For this review, take the finished solid that the model builds, in its own axes (mm). Face numbers are marked on the shaded views. A direction names the side the tool comes from. Round coordinates to 2 decimals unless told otherwise and drop trailing zeros. Write each loop counter-clockwise with the first axis right and the second up, starting at its lowest first coordinate (ties: lowest second). Pieces come first, ordered by that corner, then holes. Notation, with made-up numbers: (1, 30.5) -> (21, 30.5) arc R12 ccw to (21, 46.5) -> close; hole circle Ø10 at (-3, -32). An arc over 180 degrees is marked (long way). Answer in a Markdown table with one row per item.
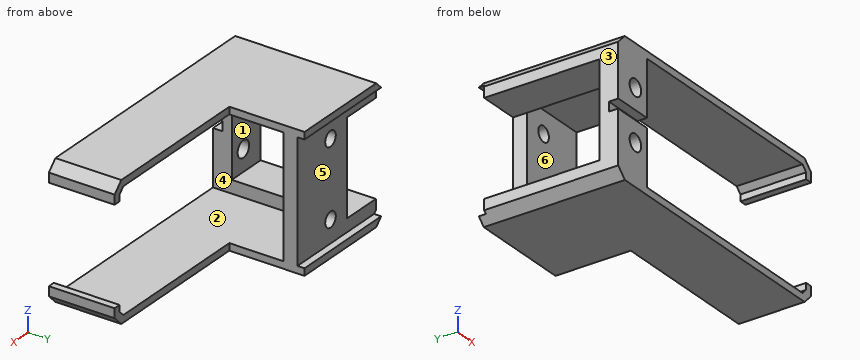
from build123d import *

# Parameters (mm, degrees)
SZKIC1_W                      = 8.7
SZKIC1_H                      = 9
SZKIC1_R                      = 1.75
DODANIE_WYCI_GNI_CIE1_DEPTH   = 2
DODANIE_WYCI_GNI_CIE1_2_DEPTH = 2
SZKIC2_W                      = 8.7
SZKIC2_H                      = 20
SZKIC2_R                      = 1.75
DODANIE_WYCI_GNI_CIE2_DEPTH   = 2
DODANIE_WYCI_GNI_CIE3_DEPTH   = 14
WYTNIJ_WYCI_GNI_CIE1_REACH    = 46.443
DODANIE_WYCI_GNI_CIE7_DEPTH   = 14.5
SZKIC10_W                     = 15
SZKIC10_H                     = 25.5
SZKIC10_R                     = 1.6
DODANIE_WYCI_GNI_CIE9_DEPTH   = 3
DODANIE_WYCI_GNI_CIE10_DEPTH  = 1.5


with BuildPart() as part:
    # Szkic1 → Dodanie-wyci_gni_cie1 (new body)
    with BuildSketch(Plane(origin=(0, 0, 0), x_dir=(1, 0, 0), z_dir=(0, 1, 0))):
        with Locations((-35.35, 5.5)):
            Rectangle(SZKIC1_W, SZKIC1_H)
        with Locations(Location((-34.5, 5.45, 0), (0, 0, 270))):
            Circle(SZKIC1_R, mode=Mode.SUBTRACT)
    extrude(amount=DODANIE_WYCI_GNI_CIE1_DEPTH)



with BuildPart() as body_2:
    # Szkic1 → Dodanie-wyci_gni_cie1 2 (new body)
    with BuildSketch(Plane(origin=(0, 0, 0), x_dir=(1, 0, 0), z_dir=(0, 1, 0))):
        with Locations((-35.35, -5.5)):
            Rectangle(SZKIC1_W, SZKIC1_H)
        with Locations(Location((-34.5, -5.45, 0), (0, 0, 90))):
            Circle(SZKIC1_R, mode=Mode.SUBTRACT)
    extrude(amount=DODANIE_WYCI_GNI_CIE1_2_DEPTH)


with BuildPart() as part_1:
    add(part.part)

    add(body_2.part)  # Dodanie-wyci_gni_cie2 merges body 2
    # Szkic2 → Dodanie-wyci_gni_cie2 (add)
    with BuildSketch(Plane(origin=(0, 2, 0), x_dir=(1, 0, 0), z_dir=(0, 1, 0))):
        with Locations((-35.35, 0)):
            Rectangle(SZKIC2_W, SZKIC2_H)
        with Locations(Location((-34.5, 5.45, 0), (0, 0, 270))):
            Circle(SZKIC2_R, mode=Mode.SUBTRACT)
        with Locations(Location((-34.5, -5.45, 0), (0, 0, 90))):
            Circle(SZKIC2_R, mode=Mode.SUBTRACT)
    extrude(amount=DODANIE_WYCI_GNI_CIE2_DEPTH)

    # Szkic5 → Dodanie-wyci_gni_cie3 (add)
    with BuildSketch(Plane(origin=(0, 0, 0), x_dir=(-1, 0, 0), z_dir=(0, -1, 0))):
        Polygon((39.7, -10), (39.7, -12.25), (37.7, -14.25), (-16.7, -14.25), (-18.7, -12.25), (-18.7, -10.25), (31, -10.25), (31, -10), align=None)
        Polygon((39.7, 10), (39.7, 12.25), (37.7, 14.25), (-16.7, 14.25), (-18.7, 12.25), (-18.7, 10.25), (31, 10.25), (31, 10), align=None)
    extrude(amount=-DODANIE_WYCI_GNI_CIE3_DEPTH)

    # Szkic7 → Wytnij-wyci_gni_cie1 (cut, up to next)
    with BuildSketch(Plane(origin=(0, 14, 0), x_dir=(1, 0, 0), z_dir=(0, 1, 0)), mode=Mode.PRIVATE) as wytnij_wyci_gni_cie1_sk1:
        Polygon((-31, 10.25), (17.2, 10.25), (17.2, 11.628679656), (16.078679656, 12.75), (-31, 12.75), align=None)
    wytnij_wyci_gni_cie1_tool1 = extrude(wytnij_wyci_gni_cie1_sk1.sketch, amount=-WYTNIJ_WYCI_GNI_CIE1_REACH, mode=Mode.PRIVATE) & part_1.part
    # Szkic7 → Wytnij-wyci_gni_cie1 (cut, up to next)
    with BuildSketch(Plane(origin=(0, 14, 0), x_dir=(1, 0, 0), z_dir=(0, 1, 0)), mode=Mode.PRIVATE) as wytnij_wyci_gni_cie1_sk2:
        Polygon((16.078679656, -12.75), (-31, -12.75), (-31, -10.25), (17.2, -10.25), (17.2, -11.628679656), align=None)
    wytnij_wyci_gni_cie1_tool2 = extrude(wytnij_wyci_gni_cie1_sk2.sketch, amount=-WYTNIJ_WYCI_GNI_CIE1_REACH, mode=Mode.PRIVATE) & part_1.part
    add(wytnij_wyci_gni_cie1_tool1.solids().sort_by_distance((-7.024435, 14, -11.495405))[0], mode=Mode.SUBTRACT)
    add(wytnij_wyci_gni_cie1_tool2.solids().sort_by_distance((-7.024435, 14, 11.495405))[0], mode=Mode.SUBTRACT)

    # Szkic8 → Dodanie-wyci_gni_cie7 (add)
    with BuildSketch(Plane(origin=(0, 14, 0), x_dir=(1, 0, 0), z_dir=(0, 1, 0))):
        Polygon((-31, 10), (-39.7, 10), (-39.7, 12.25), (-37.7, 14.25), (-16, 14.25), (-16, 12.75), (-31, 12.75), align=None)
        Polygon((-16, -12.75), (-31, -12.75), (-31, -10), (-39.7, -10), (-39.7, -12.25), (-37.7, -14.25), (-16, -14.25), align=None)
    extrude(amount=DODANIE_WYCI_GNI_CIE7_DEPTH)

    # Szkic10 → Dodanie-wyci_gni_cie9 (add)
    with BuildSketch(Plane(origin=(0, 28.5, 0), x_dir=(1, 0, 0), z_dir=(0, 1, 0))):
        with Locations((-23.5, 0)):
            Rectangle(SZKIC10_W, SZKIC10_H)
        with Locations(Location((-26, 8, 0), (0, 0, 270))):
            Circle(SZKIC10_R, mode=Mode.SUBTRACT)
        with Locations(Location((-26, -8, 0), (0, 0, 90))):
            Circle(SZKIC10_R, mode=Mode.SUBTRACT)
    extrude(amount=-DODANIE_WYCI_GNI_CIE9_DEPTH)

    # Szkic11 → Dodanie-wyci_gni_cie10 (add)
    with BuildSketch(Plane(origin=(0, 28.5, 0), x_dir=(1, 0, 0), z_dir=(0, 1, 0))):
        Polygon((-16, 12.75), (-16, 14.25), (-37.7, 14.25), (-39.2, 12.75), align=None)
        Polygon((-37.7, -14.25), (-39.2, -12.75), (-16, -12.75), (-16, -14.25), align=None)
    extrude(amount=DODANIE_WYCI_GNI_CIE10_DEPTH)


solid = part_1.part
1) Consider section D-D on x = 2.5. State the section outline as (y, z) points.
Solved:
| item | result |
|---|---|
| outline | (0, -14.25) -> (14, -14.25) -> (14, -12.75) -> (0, -12.75) -> close; (0, 12.75) -> (14, 12.75) -> (14, 14.25) -> (0, 14.25) -> close |
2) For line 1 (Z direction, x = -7.5, y = 12.5); line 2 (X direction, y = 1.4, z = -5.45); line 3 (X direction, y = 26.25, z = -10.25), list the stretches that pass through material, from the lowest coordinate up. Write a range as [from, to].
Solved:
| item | result |
|---|---|
| line 1 | [-14.25, -12.75], [12.75, 14.25] |
| line 2 | [-39.7, -36.25], [-32.75, -31] |
| line 3 | [-39.7, -16] |
3) Clearance check with flat-ended pins moving along their axes: pin 1 Ø4.5 at (x, z) = (-25.5, -5) entering from -Y; pin 2 Ø1.5 at (y, z) = (27, 4.5) entering from -X; pin 3 Ø3 at (x, z) = (-26, -8) entering from -Y; pin 4 Ø7.5 at (x, y) = (-5.5, 17.5) entering from -Z. State where each tip first meets the part, or that it passes through.
Solved:
| item | result |
|---|---|
| pin 1 | y = 25.5 |
| pin 2 | x = -31 |
| pin 3 | through |
| pin 4 | z = -14.25 |
4) Consider section C-C on z = -8. State the section outline as (x, y) points.
Solved:
| item | result |
|---|---|
| outline | (-39.7, 0) -> (-31, 0) -> (-31, 4) -> (-39.7, 4) -> close; (-31, 25.5) -> (-27.6, 25.5) -> (-27.6, 28.5) -> (-31, 28.5) -> close; (-24.4, 25.5) -> (-16, 25.5) -> (-16, 28.5) -> (-24.4, 28.5) -> close |
5) Mouldability with a two-part tool opening along X and no side actions: class the marked faces 1, 2 and 3 as pulls with the +X half, pulls with the -X half, needs draft (parallel to the pull), parting line crosses it, or undercut.
Solved:
| item | result |
|---|---|
| face 1 | needs draft |
| face 2 | undercut |
| face 3 | pulls with the -X half |
6) Consider section B-B on y = 11. State the section outline as (x, z) points, then the cut area to 3 significant figures.
Solved:
| item | result |
|---|---|
| outline | (-39.7, -12.25) -> (-37.7, -14.25) -> (16.7, -14.25) -> (18.7, -12.25) -> (18.7, -10.25) -> (17.2, -10.25) -> (17.2, -11.63) -> (16.08, -12.75) -> (-31, -12.75) -> (-31, -10) -> (-39.7, -10) -> close; (-39.7, 10) -> (-31, 10) -> (-31, 12.75) -> (16.08, 12.75) -> (17.2, 11.63) -> (17.2, 10.25) -> (18.7, 10.25) -> (18.7, 12.25) -> (16.7, 14.25) -> (-37.7, 14.25) -> (-39.7, 12.25) -> close |
| area | 224 mm² |
7) For the marked faces 4, 5 and 6, list the 3-axis set-ups (+Z, -Z, +X, -X, +Y, -Y) from which the entire face can be reached by the end or side of a thin tool; tool diameter is ignored.
Solved:
| item | result |
|---|---|
| face 4 | -Y |
| face 5 | +X, -X, +Y |
| face 6 | +X, -Y |
8) Consider section A-A on x = -26. State the section outline as (y, z) points.
Solved:
| item | result |
|---|---|
| outline | (0, -14.25) -> (30, -14.25) -> (30, -12.75) -> (28.5, -12.75) -> (28.5, -9.6) -> (25.5, -9.6) -> (25.5, -12.75) -> (0, -12.75) -> close; (0, 12.75) -> (25.5, 12.75) -> (25.5, 9.6) -> (28.5, 9.6) -> (28.5, 12.75) -> (30, 12.75) -> (30, 14.25) -> (0, 14.25) -> close; (25.5, -6.4) -> (28.5, -6.4) -> (28.5, 6.4) -> (25.5, 6.4) -> close |
